Check sheet for the modelled part. Datum: model origin and axes. Units: mm. Face numbers are marked on the shaded views. A direction names the side the tool comes from. Give positions to 0.01 mm unless a question says otherwise; leave off trailing zeros. Order: outer loops, then holes, each group sorted by start corner. A loop starts at its lowest first (then second) coordinate and runs counter-clockwise, first axis right, second up. Notation, with made-up numbers: (57.5, 26) -> (89.5, 26) arc R20 cw to (89.5, 51) -> close; hole circle Ø8 at (64.5, -23.75). An arc over 180 degrees is marked (long way). One line per question, with ' | ' between items.
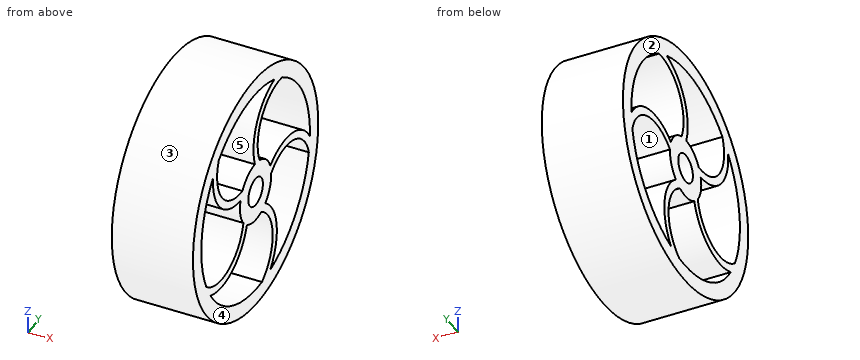
```python
from build123d import *

# Parameters (mm, degrees)
SKETCH1_R           = 3.75
SKETCH1_R_2         = 1.75
BOSS_EXTRUDE1_DEPTH = 10
SKETCH2_R           = 15
SKETCH2_R_2         = 13
BOSS_EXTRUDE2_DEPTH = 10
BOSS_EXTRUDE3_DEPTH = 10
CIRPATTERN1_COUNT   = 5


with BuildPart() as part:
    # Sketch1 → Boss-Extrude1 (new body)
    with BuildSketch(Plane(origin=(0, 0, 0), x_dir=(0, 0, -1), z_dir=(1, 0, 0))):
        Circle(SKETCH1_R)
        Circle(SKETCH1_R_2, mode=Mode.SUBTRACT)
    extrude(amount=-BOSS_EXTRUDE1_DEPTH)



with BuildPart() as body_2:
    # Sketch2 → Boss-Extrude2 (new body)
    with BuildSketch(Plane(origin=(0, 0, 0), x_dir=(0, 0, -1), z_dir=(1, 0, 0))):
        Circle(SKETCH2_R)
        Circle(SKETCH2_R_2, mode=Mode.SUBTRACT)
    extrude(amount=-BOSS_EXTRUDE2_DEPTH)


with BuildPart() as part_1:
    add(part.part)

    add(body_2.part)  # Boss-Extrude3 merges body 2
    # Sketch3 → Boss-Extrude3 (add)
    with BuildSketch(Plane(origin=(0, 0, 0), x_dir=(0, 0, -1), z_dir=(1, 0, 0))):
        with BuildLine():
            ThreePointArc((-12.185926249, 4.528046097), (-9.008421397, 0.308117229), (-3.746637972, -0.158757395))
            ThreePointArc((-3.746637972, -0.158757395), (-3.727921816, 0.406323685), (-3.624463026, 0.962168268))
            ThreePointArc((-3.624463026, 0.962168268), (-9.003588829, 1.482702332), (-11.340490704, 6.355570045))
            ThreePointArc((-11.340490704, 6.355570045), (-11.798645456, 5.458201663), (-12.185926249, 4.528046097))
        make_face()
    boss_extrude3 = extrude(amount=-BOSS_EXTRUDE3_DEPTH)

    # CirPattern1: Boss-Extrude3 ×5 about axis
    cirpattern1_axis = Axis((0, 0, 0), (1, 0, 0))
    for i in range(1, CIRPATTERN1_COUNT):
        add(boss_extrude3.rotate(cirpattern1_axis, i * 360 / CIRPATTERN1_COUNT))


solid = part_1.part
```
Q1. Section check B-B (z = -10.75). Enter the section's corners in (x, y).
Result sheet:
outline: (-10, -10.46) -> (0, -10.46) -> (0, -7.31) -> (-10, -7.31) -> close; (-10, 3.5) -> (0, 3.5) -> (0, 4.6) -> (-10, 4.6) -> close; (-10, 7.31) -> (0, 7.31) -> (0, 10.46) -> (-10, 10.46) -> close
Q2. Section check A-A (x = -1.5). Enter the section's corners in (y, z), and give its area (3 significant figures).
Result sheet:
outline: circle Ø30 at (0, 0); hole (-11.81, -5.44) arc R5.5 ccw to (-2.91, -2.37) arc R3.75 cw to (-3.61, 1.01) arc R6.5 cw to (-10.19, 8.07) arc R13 ccw to start; hole (-10.83, -7.2) arc R13 ccw to (1.52, -12.91) arc R5.5 ccw to (1.35, -3.5) arc R3.75 cw to (-2.07, -3.12) arc R6.5 cw to start; hole (-8.82, 9.55) arc R5.5 ccw to (-3.15, 2.04) arc R3.75 cw to (-0.16, 3.75) arc R6.5 cw to (4.53, 12.19) arc R13 ccw to start; hole circle Ø3.5 at (0, 0); hole (0.96, 3.62) arc R3.75 cw to (3.51, 1.31) arc R6.5 cw to (12.99, -0.54) arc R13 ccw to (6.36, 11.34) arc R5.5 ccw to start; hole (2.33, -2.94) arc R6.5 cw to (3.5, -12.52) arc R13 ccw to (12.75, -2.54) arc R5.5 ccw to (3.74, 0.2) arc R3.75 cw to start | area: 266 mm2
Q3. Section check D-D (y = 8). Enter the section's corners in (x, z).
Result sheet:
outline: (-10, -12.69) -> (0, -12.69) -> (0, -10.25) -> (-10, -10.25) -> close; (-10, 1.58) -> (0, 1.58) -> (0, 2.58) -> (-10, 2.58) -> close; (-10, 10.25) -> (0, 10.25) -> (0, 12.69) -> (-10, 12.69) -> close
Q4. Mould release check, pull along Y, two halves, no side actions. Record for the marked faces 3, 4 and 5: pulls with the +Y half, pulls with the -Y half, needs draft (parallel to the pull), parting line crosses it, or undercut.
Result sheet:
face 3: parting line crosses it | face 4: needs draft | face 5: undercut
Q5. Access from +Z, -Z, +X, -X, +Y, -Y to the whole of each face (thin tool, end or side, straight path). Record for the marked faces 1 and 2.
Result sheet:
face 1: +X, -X | face 2: +Z, -Z, -X, +Y, -Y
Q6. Thickness scan on line 1 (Y direction, x = -2, z = 0); line 2 (Y direction, x = -9.25, z = -0.25); line 3 (Z direction, x = -2.5, y = 6.75). Record the ranges inside material, lowest first.
Result sheet:
line 1: y = -15 to -13, -3.75 to -1.75, 1.75 to 3.75, 11.31 to 12.63, 13 to 15 | line 2: y = -15 to -13, -3.74 to -1.73, 1.73 to 3.74, 11.54 to 12.8, 13 to 15 | line 3: z = -13.4 to -11.11, 1.57 to 2.58, 11.11 to 13.4
Q7. Depth check by flat-ended pin: pin 1 Ø6 at (x, z) = (-8.5, 9) entering from +Y; pin 2 Ø2 at (x, z) = (-5.5, -5) entering from -Y; pin 3 Ø3 at (y, z) = (0, 0) entering from -X (3 decimals). Enter the tip coordinate at first touch or a pass-through.
Result sheet:
pin 1: stops at y = 13.75 | pin 2: stops at y = -14.46 | pin 3: passes through
Q8. Section check C-C (z = -1). Enter the section's corners in (x, y).
Result sheet:
outline: (-10, -14.97) -> (0, -14.97) -> (0, -12.96) -> (-10, -12.96) -> close; (-10, -3.61) -> (0, -3.61) -> (0, -1.44) -> (-10, -1.44) -> close; (-10, 1.44) -> (0, 1.44) -> (0, 3.61) -> (-10, 3.61) -> close; (-10, 12.1) -> (0, 12.1) -> (0, 14.97) -> (-10, 14.97) -> close
